from build123d import *

# Parameters (mm, degrees)
SKETCH1_R                      = 2.55
SKETCH1_R_2                    = 11
BASE_DEPTH                     = 5
SKETCH1_3_R                    = 15
SKETCH1_3_R_2                  = 11
STEM_DEPTH                     = 150
SKETCH4_W                      = 90.4
SKETCH4_H                      = 80
TOP_PLATE_DEPTH                = 10
SKETCH6_W                      = 90.4
SKETCH6_H                      = 10
BOSS_EXTRUDE7_DEPTH            = 19
RIB1_START                     = -2.5
RIB1_DEPTH                     = 5
CIRPATTERN6_COUNT              = 6
CUT_EXTRUDE1_REACH             = 170.039
SKETCH10_R                     = 3.05
CUT_EXTRUDE1_DIRECTION_2_DEPTH = 169.039429897
FILLET1_R                      = 10
FILLET2_R                      = 10
SKETCH11_R                     = 55
NEW_BASE_DEPTH                 = 10
RIB2_START                     = -2.5
RIB2_DEPTH                     = 5
CIRPATTERN7_COUNT              = 6
SKETCH13_R                     = 3.05
CUT_EXTRUDE2_DEPTH             = 10
FILLET3_R                      = 10
SKETCH15_R                     = 11
REMOVE_CENTER_DEPTH            = 162.573512681
BASE_CUT_DEPTH                 = 40


with BuildPart() as part:
    # Sketch1 → base (new body)
    with BuildSketch(Plane(origin=(0, 0, 0), x_dir=(1, 0, 0), z_dir=(0, 1, 0))):
        with BuildLine():
            Line((-16, 25.377155081), (-42.833333333, 8.459051694))
            ThreePointArc((-42.833333333, 8.459051694), (-47.5, 0), (-42.833333333, -8.459051694))
            Line((-42.833333333, -8.459051694), (-16, -25.377155081))
            ThreePointArc((-16, -25.377155081), (0, -30), (16, -25.377155081))
            Line((16, -25.377155081), (42.833333333, -8.459051694))
            ThreePointArc((42.833333333, -8.459051694), (47.5, 0), (42.833333333, 8.459051694))
            Line((42.833333333, 8.459051694), (16, 25.377155081))
            ThreePointArc((16, 25.377155081), (0, 30), (-16, 25.377155081))
        make_face()
        with Locations(Location((-37.5, 0, 0), (0, 0, 270))):
            Circle(SKETCH1_R, mode=Mode.SUBTRACT)
        with Locations(Location((37.5, 0, 0), (0, 0, 270))):
            Circle(SKETCH1_R, mode=Mode.SUBTRACT)
        with Locations(Location((0, 0, 0), (0, 0, 270))):
            Circle(SKETCH1_R_2, mode=Mode.SUBTRACT)
    extrude(amount=BASE_DEPTH)

    # Sketch1<3> → stem (add)
    with BuildSketch(Plane(origin=(0, 0, 0), x_dir=(1, 0, 0), z_dir=(0, 1, 0))):
        with Locations(Location((0, 0, 0), (0, 0, 270))):
            Circle(SKETCH1_3_R)
        with Locations(Location((0, 0, 0), (0, 0, 270))):
            Circle(SKETCH1_3_R_2, mode=Mode.SUBTRACT)
    extrude(amount=STEM_DEPTH)

    # Sketch4 → top plate (add)
    with BuildSketch(Plane(origin=(0, 150, 0), x_dir=(1, 0, 0), z_dir=(0, 1, 0))):
        Rectangle(SKETCH4_W, SKETCH4_H)
    extrude(amount=-TOP_PLATE_DEPTH)

    # Sketch6 → Boss-Extrude7 (add)
    with BuildSketch(Plane.XY.offset(40)):
        with Locations((0, 145)):
            Rectangle(SKETCH6_W, SKETCH6_H)
    extrude(amount=BOSS_EXTRUDE7_DEPTH)

    # Rib1: read off the stored shape, not the designer's step
    # Rib1 outline → Rib1 (add)
    with BuildSketch(Plane(origin=(0, 0, 0), x_dir=(0, 0, -1), z_dir=(1, 0, 0)).offset(RIB1_START)):
        Polygon((-15, 110), (-14.790199458, 110), (-14.790199458, 140), (-40, 140), align=None)
    rib1 = extrude(amount=RIB1_DEPTH)

    # CirPattern6: Rib1 ×6 about axis
    cirpattern6_axis = Axis((0, 0, 0), (0, 1, 0))
    for i in range(1, CIRPATTERN6_COUNT):
        add(rib1.rotate(cirpattern6_axis, i * 360 / CIRPATTERN6_COUNT))

    # Sketch10 → Cut-Extrude1 (cut, up to next)
    with BuildSketch(Plane(origin=(0, 150, 0), x_dir=(1, 0, 0), z_dir=(0, 1, 0)), mode=Mode.PRIVATE) as cut_extrude1_sk1:
        with Locations(Location((35.2, -49, 0), (0, 0, 90))):
            Circle(SKETCH10_R)
    cut_extrude1_tool1 = extrude(cut_extrude1_sk1.sketch, amount=-CUT_EXTRUDE1_REACH, mode=Mode.PRIVATE) & part.part
    # Sketch10 → Cut-Extrude1 (cut, up to next)
    with BuildSketch(Plane(origin=(0, 150, 0), x_dir=(1, 0, 0), z_dir=(0, 1, 0)), mode=Mode.PRIVATE) as cut_extrude1_sk2:
        with Locations(Location((-35.2, -49, 0), (0, 0, 90))):
            Circle(SKETCH10_R)
    cut_extrude1_tool2 = extrude(cut_extrude1_sk2.sketch, amount=-CUT_EXTRUDE1_REACH, mode=Mode.PRIVATE) & part.part
    add(cut_extrude1_tool1.solids().sort_by_distance((35.2, 150, 49))[0], mode=Mode.SUBTRACT)
    add(cut_extrude1_tool2.solids().sort_by_distance((-35.2, 150, 49))[0], mode=Mode.SUBTRACT)

    # Sketch10 → Cut-Extrude1 direction 2 (cut)
    with BuildSketch(Plane(origin=(0, 150, 0), x_dir=(1, 0, 0), z_dir=(0, 1, 0))):
        with Locations(Location((35.2, -49, 0), (0, 0, 90))):
            Circle(SKETCH10_R)
        with Locations(Location((-35.2, -49, 0), (0, 0, 90))):
            Circle(SKETCH10_R)
    extrude(amount=CUT_EXTRUDE1_DIRECTION_2_DEPTH, mode=Mode.SUBTRACT)

    # Fillet1
    fillet1_edges = [part.edges().sort_by_distance(p)[0] for p in [
        (-45.2, 145, 59),
    ]]
    fillet(fillet1_edges, radius=FILLET1_R)

    # Fillet2
    fillet2_edges = [part.edges().sort_by_distance(p)[0] for p in [
        (45.2, 145, 59),
    ]]
    fillet(fillet2_edges, radius=FILLET2_R)

    # Sketch11 → new base (add)
    with BuildSketch(Plane.XZ):
        with Locations(Location((0, 0, 0), (0, 0, 270))):
            Circle(SKETCH11_R)
    extrude(amount=-NEW_BASE_DEPTH)

    # Rib2: read off the stored shape, not the designer's step
    # Rib2 outline → Rib2 (add)
    with BuildSketch(Plane.XY.offset(RIB2_START)):
        Polygon((13, 10), (55, 10), (13, 52), align=None)
    rib2 = extrude(amount=RIB2_DEPTH)

    # CirPattern7: Rib2 ×6 about axis
    cirpattern7_axis = Axis((0, 0, 0), (0, 1, 0))
    for i in range(1, CIRPATTERN7_COUNT):
        add(rib2.rotate(cirpattern7_axis, i * 360 / CIRPATTERN7_COUNT))

    # Sketch13 → Cut-Extrude2 (cut)
    with BuildSketch(Plane.XZ):
        with Locations(Location((-37.5, -25, 0), (0, 0, 270))):
            Circle(SKETCH13_R)
        with Locations(Location((-37.5, 25, 0), (0, 0, 270))):
            Circle(SKETCH13_R)
        with Locations(Location((37.5, 25, 0), (0, 0, 270))):
            Circle(SKETCH13_R)
        with Locations(Location((37.5, -25, 0), (0, 0, 270))):
            Circle(SKETCH13_R)
    extrude(amount=-CUT_EXTRUDE2_DEPTH, mode=Mode.SUBTRACT)

    # Fillet3
    fillet3_edges = [part.edges().sort_by_distance(p)[0] for p in [
        (45.2, 145, -40),
        (-45.2, 145, -40),
    ]]
    fillet(fillet3_edges, radius=FILLET3_R)

    # Sketch15 → remove center (cut, through all)
    with BuildSketch(Plane(origin=(0, 10, 0), x_dir=(1, 0, 0), z_dir=(0, 1, 0))):
        with Locations(Location((0, 0, 0), (0, 0, 270))):
            Circle(SKETCH15_R)
    extrude(amount=-REMOVE_CENTER_DEPTH, mode=Mode.SUBTRACT)

    # Sketch16 → base cut (cut)
    with BuildSketch(Plane.XZ):
        with BuildLine():
            Line((-37.749172176, 40), (37.749172176, 40))
            ThreePointArc((37.749172176, 40), (0, 55), (-37.749172176, 40))
        make_face()
        with BuildLine():
            ThreePointArc((-37.749172176, -40), (0, -55), (37.749172176, -40))
            Line((37.749172176, -40), (-37.749172176, -40))
        make_face()
    extrude(amount=-BASE_CUT_DEPTH, mode=Mode.SUBTRACT)


with BuildPart() as base_cut_kept_piece:
    # of the separate pieces the step leaves, the one the design keeps (base_cut_pieces_kept)
    add(part.part.solids().sort_by_distance((45.2, 140, -30))[0])


solid = base_cut_kept_piece.part
For this review, take the finished solid that the model builds, in its own axes (mm). A direction names the side the tool comes from. Give positions to 0.01 mm unless a question says otherwise; leave off trailing zeros. Order: outer loops, then holes, each group sorted by start corner. A loop starts at its lowest first (then second) coordinate and runs counter-clockwise, first axis right, second up. Notation, with made-up numbers: M 31.25,-2 L 59.25,-2 A14 cw 59.25,25 Z; hole C -7,58 d2. An arc over 180 degrees is marked long. Answer in a Markdown table with one row per item. Add a question column.
(1) Consider section C-C on x = -7.5. State the section outline as (y, z) points.
(2) For pin 1 (12 mm diameter, centred on x = 16, z = 47, fed in from -Y); pin 2 (6 mm diameter, centred on y = 129, z = -23, fed in from +X); pin 3 (8 mm diameter, centred on x = -31.5, z = -12, fed in from -Y); pin 4 (1.5 mm diameter, centred on y = 80, z = 7.5, fed in from +X), all flat-tipped, find the tip position at first contact; note any pin that passes through.
(3) Consider section A-A on z = -26. State the section outline as (x, y) points, and give its area (3 significant figures).
(4) Consider section B-B on y = 124.5. State the section outline as (x, z) points, and give its area (3 significant figures).
(5) Consider section D-D on y = 106.5. State the section outline as (x, z) points, and give its area (3 significant figures).
(6) Wall thickness on probe 1 along Z at (x, y) = (37, 8); probe 2 along Z at (x, y) = (-35.2, 143.25); probe 3 along X at (y, z) = (4, -25): over which ranges is each line inside the solid? List them lowest first. Write a range as [from, to].
(7) Mouldability with a two-part tool opening along Z and no side actions: class faces 1 (the face through (-35, 30, 0)), 2 (the face through (-32.223, 145.07, 49.661)), 3 (the face through (-15.69, 33.559, 27.246)) as +Z half, -Z half, draft (parallel to the pull), parting line (faces both ways), or undercut.
(8) For faces 4 (the face through (0.035, 125.21, -27.675)), 5 (the face through (-26, 21, 2.5)), 6 (the face through (15.75, 33.56, 27.21)), 7 (the face through (54.996, 4.93, -0.627)), 8 (the face through (-10.95, 25.919, 23.965)), list the 3-axis set-ups (+Z, -Z, +X, -X, +Y, -Y) from which the entire face can be reached by the end or side of a thin tool; tool diameter is ignored.
Evaluation:
| question | item | result |
|---|---|---|
| 1 | outline | M 0,-40 L 10,-40 L 10,-17.99 L 45.67,-17.99 L 50,-12.99 L 140,-12.99 L 140,-40 L 150,-40 L 150,59 L 140,59 L 140,12.99 L 50,12.99 L 45.67,17.99 L 10,17.99 L 10,40 L 0,40 L 0,8.05 L 140,8.05 L 140,-8.05 L 0,-8.05 Z |
| 2 | pin 1 | stops at y = 140 |
| 2 | pin 2 | stops at x = 2.5 |
| 2 | pin 3 | stops at y = 0 |
| 2 | pin 4 | stops at x = 13.4 |
| 3 | outline | M -48.47,0 L -40.38,0 L -40.38,10 L -48.47,10 Z; M -45.2,140 L -2.5,140 L -2.5,123.2 L 2.5,123.2 L 2.5,140 L 45.2,140 L 45.2,150 L -45.2,150 Z; M -34.62,0 L 34.62,0 L 34.62,10 L 17.9,10 L 17.9,33.53 L 12.12,36.42 L 12.12,10 L -12.12,10 L -12.12,36.42 L -17.9,33.53 L -17.9,10 L -34.62,10 Z; M 40.38,0 L 48.47,0 L 48.47,10 L 40.38,10 Z |
| 3 | area | 2,130 mm^2 |
| 4 | outline | M -24.7,-11.38 L -22.2,-15.71 L -11.56,-9.56 A15 ccw -2.5,-14.79 L -2.5,-27.08 L 2.5,-27.08 L 2.5,-14.79 A15 ccw 11.56,-9.56 L 22.2,-15.71 L 24.7,-11.38 L 14.06,-5.23 A15 ccw 14.06,5.23 L 24.7,11.38 L 22.2,15.71 L 11.56,9.56 A15 ccw 2.5,14.79 L 2.5,27.08 L -2.5,27.08 L -2.5,14.79 A15 ccw -11.56,9.56 L -22.2,15.71 L -24.7,11.38 L -14.06,5.23 A15 ccw -14.06,-5.23 Z; hole C 0,0 d22 |
| 4 | area | 691 mm^2 |
| 5 | outline | C 0,0 d30; hole C 0,0 d22 |
| 5 | area | 327 mm^2 |
| 6 | probe 1 | z = [-40, -28.01], [-21.99, 21.99], [28.01, 40] |
| 6 | probe 2 | z = [-40, 45.95], [52.05, 59] |
| 6 | probe 3 | x = [-48.99, -40.55], [-34.45, 34.45], [40.55, 48.99] |
| 7 | face 1 | draft |
| 7 | face 2 | undercut |
| 7 | face 3 | +Z half |
| 8 | face 4 | -Z, +X, -X |
| 8 | face 5 | -X |
| 8 | face 6 | +Z, +X |
| 8 | face 7 | +X, -Y |
| 8 | face 8 | +Z |
